from build123d import *

# Parameters (mm, degrees)
F1_DEPTH  = 18.288
F3_W      = 38.6883560568
F3_H      = 14.0357739292
F4_DEPTH  = 35.56
F5_R      = 6.7564
F6_R      = 6.7453126933
F9_DEPTH  = 51.562
F11_R     = 3.3108000024
F12_DEPTH = 139.954


with BuildPart() as f1:
    # F0 (on Top) → F1 (new body)
    with BuildSketch(Plane.XY):
        with BuildLine():
            Line((37.3380035162, 16.6687499732), (-35.0043773651, 16.6687499732))
            Line((-35.0043773651, 16.6687499732), (-35.0043773651, 16.4739897927))
            ThreePointArc((-35.0043773651, 16.4739897927), (-22.7661779649, 11.4047616221), (-17.6969497944, -0.8334377781))
            ThreePointArc((-17.6969497944, -0.8334377781), (-22.7661779649, -13.0716371782), (-35.0043773651, -18.1408653488))
            Line((-35.0043773651, -18.1408653488), (-35.0043773651, -18.3356255293))
            Line((-35.0043773651, -18.3356255293), (37.3380035162, -18.3356255293))
            Line((37.3380035162, -18.3356255293), (37.3380035162, -18.0797577525))
            ThreePointArc((37.3380035162, -18.0797577525), (20.0916835417, -0.8334377781), (37.3380035162, 16.4128821964))
            Line((37.3380035162, 16.4128821964), (37.3380035162, 16.6687499732))
        make_face()
        with BuildLine():
            ThreePointArc((54.5843234907, -0.8334377781), (49.5329933207, 11.3615520264), (37.3380035162, 16.4128821964))
            Line((37.3380035162, 16.4128821964), (37.3380035162, 6.7044516866))
            ThreePointArc((37.3380035162, 6.7044516866), (42.6680962725, 4.4966549783), (44.8758929809, -0.8334377781))
            ThreePointArc((44.8758929809, -0.8334377781), (42.6680962725, -6.1635305344), (37.3380035162, -8.3713272428))
            Line((37.3380035162, -8.3713272428), (37.3380035162, -18.0797577525))
            ThreePointArc((37.3380035162, -18.0797577525), (49.5329933207, -13.0284275825), (54.5843234907, -0.8334377781))
        make_face()
        with BuildLine():
            Line((-35.0043773651, 5.5813243756), (-35.0043773651, 16.4739897927))
            ThreePointArc((-35.0043773651, 16.4739897927), (-52.3118049358, -0.8334377781), (-35.0043773651, -18.1408653488))
            Line((-35.0043773651, -18.1408653488), (-35.0043773651, -7.2481999317))
            ThreePointArc((-35.0043773651, -7.2481999317), (-41.4191395188, -0.8334377781), (-35.0043773651, 5.5813243756))
        make_face()
        with BuildLine():
            ThreePointArc((-17.6969497944, -0.8334377781), (-22.7661779649, 11.4047616221), (-35.0043773651, 16.4739897927))
            Line((-35.0043773651, 16.4739897927), (-35.0043773651, 5.5813243756))
            ThreePointArc((-35.0043773651, 5.5813243756), (-30.4684555466, 3.7024840405), (-28.5896152114, -0.8334377781))
            ThreePointArc((-28.5896152114, -0.8334377781), (-30.4684555466, -5.3693595966), (-35.0043773651, -7.2481999317))
            Line((-35.0043773651, -7.2481999317), (-35.0043773651, -18.1408653488))
            ThreePointArc((-35.0043773651, -18.1408653488), (-22.7661779649, -13.0716371782), (-17.6969497944, -0.8334377781))
        make_face()
        with BuildLine():
            Line((37.3380035162, 6.7044516866), (37.3380035162, 16.4128821964))
            ThreePointArc((37.3380035162, 16.4128821964), (20.0916835417, -0.8334377781), (37.3380035162, -18.0797577525))
            Line((37.3380035162, -18.0797577525), (37.3380035162, -8.3713272428))
            ThreePointArc((37.3380035162, -8.3713272428), (29.8001140515, -0.8334377781), (37.3380035162, 6.7044516866))
        make_face()
    extrude(amount=F1_DEPTH)

    # F3 (on offset) → F4 (join)
    with BuildSketch(Plane.XY.offset(18.288)):
        with Locations((1.2210039422, 0.1680313144)):
            Rectangle(F3_W, F3_H)
    extrude(amount=F4_DEPTH)

    # F5
    f5_edges = [f1.edges().sort_by_distance(p)[0] for p in [
        (1.221004, -6.849856, 53.848),
    ]]
    fillet(f5_edges, radius=F5_R)

    # F6
    f6_edges = [f1.edges().sort_by_distance(p)[0] for p in [
        (1.221004, 7.185918, 53.848),
    ]]
    fillet(f6_edges, radius=F6_R)

    # F8 (on offset) → F9 (cut)
    with BuildSketch(Plane.XZ.offset(14.732)):
        with BuildLine():
            Line((5.6341080926, 53.8724064827), (-5.0880652852, 53.8724064827))
            Line((-5.0880652852, 53.8724064827), (-5.0880652852, 31.7973420024))
            Line((-5.0880652852, 31.7973420024), (-5.034370235, 31.7973420024))
            ThreePointArc((-5.034370235, 31.7973420024), (0.2730214037, 37.1047336411), (5.5804130424, 31.7973420024))
            Line((5.5804130424, 31.7973420024), (5.6341080926, 31.7973420024))
            Line((5.6341080926, 31.7973420024), (5.6341080926, 53.8724064827))
        make_face()
        with BuildLine():
            ThreePointArc((5.5804130424, 31.7973420024), (0.2730214037, 37.1047336411), (-5.034370235, 31.7973420024))
            Line((-5.034370235, 31.7973420024), (5.5804130424, 31.7973420024))
        make_face()
        with BuildLine():
            Line((5.5804130424, 31.7973420024), (-5.034370235, 31.7973420024))
            ThreePointArc((-5.034370235, 31.7973420024), (0.2730214037, 26.4899503636), (5.5804130424, 31.7973420024))
        make_face()
    extrude(amount=-F9_DEPTH, mode=Mode.SUBTRACT)

    # F11 (on offset) → F12 (cut)
    with BuildSketch(Plane.YZ.offset(25.4)):
        with Locations((0, 47.6729050279)):
            Circle(F11_R)
    extrude(amount=-F12_DEPTH, mode=Mode.SUBTRACT)


solid = f1.part
Verification items for the finished model (mm, model axes). A direction names the side the tool comes from. Coordinates: 2 decimals unless noted, no trailing zeros. Order: outer loops, then holes, each group sorted by start corner. A loop starts at its lowest first (then second) coordinate and runs counter-clockwise, first axis right, second up. Notation, with made-up numbers: M 38.25,49 L 89.25,49 A18 ccw 89.25,57 Z; hole C -4.75,-25.75 d6. An arc over 180 degrees is marked long. One line per item, written item: value. Start each with the question number.
Item 1: Mould release check, pull along X, two halves, no side actions. Record for faces 6 (the flat face through (0, -1, 0)), 7 (the flat face through (20.565, 0, 36)), 8 (the flat face through (-5.088, 0, 41)): released by +X, released by -X, zero draft, split by the parting line, or undercut.
Item 2: Sectioned sample at C-C (z = 38). Enter the section's corners in (x, y).
Item 3: Access from +Z, -Z, +X, -X, +Y, -Y to the whole of each face (thin tool, end or side, straight path). Record for faces 1 (the cylindrical face through (13.2, -0.72, 44.44)), 2 (the flat face through (-18.123, 0, 36)), 3 (the flat face through (5, -6.85, 29)), 4 (the flat face through (5.634, 0, 40)), 5 (the flat face through (5, 7.186, 29)).
Item 4: Gauge pin test, flat ends, axial feed: pin 1 (1.5 mm diameter, centred on x = 29, y = 12.5, fed in from -Z); pin 2 (3 mm diameter, centred on y = 7, z = 40, fed in from +X); pin 3 (1.5 mm diameter, centred on y = -2.5, z = 17.5, fed in from -X); pin 4 (2 mm diameter, centred on x = -21, y = -8.5, fed in from +Z). Record the tip position at first contact, or that the pin passes through.
Item 5: Sectioned sample at B-B (x = 43.5). Enter the section's corners in (y, z).
Item 6: Scan lines: probe 1 along Z at (x, y) = (17, 0); probe 2 along X at (y, z) = (0.5, 4.5); probe 3 along X at (y, z) = (-3.5, 46). Record each from-to range of solid material in increasing order.
Item 7: Sectioned sample at D-D (x = 12). Enter the section's corners in (y, z), then the cut area to 3 significant figures.
Conclusion:
1. face 6: zero draft
1. face 7: released by +X
1. face 8: undercut
2. outline: M -18.12,-6.85 L -5.09,-6.85 L -5.09,7.19 L -18.12,7.19 Z; M 5.63,-6.85 L 20.57,-6.85 L 20.57,7.19 L 5.63,7.19 Z
3. face 1: +X, -X
3. face 2: +Z, -X, +Y, -Y
3. face 3: +Z, +X, -X, -Y
3. face 4: +Z, +Y, -Y
3. face 5: +Z, +X, -X, +Y
4. pin 1: stops at z = 0
4. pin 2: stops at x = 20.57
4. pin 3: stops at x = -52.29
4. pin 4: stops at z = 18.29
5. outline: M -16.94,0 L -5.18,0 L -5.18,18.29 L -16.94,18.29 Z; M 3.51,0 L 15.27,0 L 15.27,18.29 L 3.51,18.29 Z
6. probe 1: z = 0 to 44.36, 50.98 to 53.85
6. probe 2: x = -52.26 to -41.28, -28.73 to 29.92, 44.76 to 54.53
6. probe 3: x = -18.12 to -5.09, 5.63 to 20.57
7. outline: M -18.34,0 L 16.67,0 L 16.67,18.29 L 7.19,18.29 L 7.19,47.1 A6.75 ccw 0.44,53.85 L -0.09,53.85 A6.76 ccw -6.85,47.09 L -6.85,18.29 L -18.34,18.29 Z; hole C 0,47.67 d6.62
7. area: 1,090 mm^2
